Here's how the part is built. I have some questions about the finished solid (model axes, mm). Coordinates: 2 decimals unless noted, no trailing zeros. Write each loop counter-clockwise with the first axis right and the second up, starting at its lowest first coordinate (ties: lowest second). Pieces come first, ordered by that corner, then holes. Notation, with made-up numbers: (64.5, 74.5) -> (73.5, 74.5) arc R17 cw to (73.5, 78.5) -> close; hole circle Ø5 at (11.5, -13.75). An arc over 180 degrees is marked (long way). Use a Markdown table: item, result. Add a question column.
Autodesk Inventor part; units mm, degrees
ref_plane "YZ Plane" through (0, 0, 0) normal (1, 0, 0) x (0, 1, 0)
ref_plane "XZ Plane" through (0, 0, 0) normal (0, 1, 0) x (-1, 0, 0)
ref_plane "XY Plane" through (0, 0, 0) normal (0, 0, 1) x (1, 0, 0)
sketch "Sketch1" plane through (0, 0, 0) normal (0, 0, 1) x (1, 0, 0)
  line L0 (19.05, -25.4) -> (-19.05, -25.4)
  line L1 (-19.05, -25.4) -> (-19.05, 25.4)
  line L2 (-19.05, 25.4) -> (19.05, 25.4)
  line L3 (19.05, 25.4) -> (19.05, -25.4)
  line L4 (19.05, -25.4) -> (-19.05, 25.4) construction
  line L5 (-19.05, -25.4) -> (19.05, 25.4) construction
  point P0 (0, 0)
  dimension "d0" = 38.1
  dimension "d1" = 50.8
extrude "Extrusion1" add sketch "Sketch1" along normal blind 6.35
chamfer "Chamfer1" distance 12.7 angle 45 2 edges at (19.05, -25.4, 3.175) (-19.05, -25.4, 3.175)
sketch "Sketch2" plane through (0, 0, 6.35) normal (0, 0, 1) x (1, 0, 0)
  line L0 (-19.05, 25.4) -> (-19.05, -12.7) construction
  line L1 (19.05, -12.7) -> (19.05, 25.4) construction
  line L2 (-19.05, -12.7) -> (19.05, -12.7) construction
  line L3 (-6.35, -25.4) -> (6.35, -25.4) construction
  line L4 (0, -25.4) -> (0, 0) construction
  circle A0 centre (0, -12.7) radius 7.1
  circle A1 centre (0, -12.7) radius 17.5 construction
  circle A2 centre (-15.875, 0.635) radius 2.1
  circle A3 centre (-15.875, 13.335) radius 2
  circle A4 centre (15.875, 0.635) radius 2.1
  circle A5 centre (15.875, 13.335) radius 2
  dimension "d7" = 14.2
  dimension "d8" = 12.7
  dimension "d9" = 35
  dimension "d10" = 4.2
  dimension "d11" = 13.335
  dimension "d12" = 3.175
  dimension "d13" = 4
  dimension "d14" = 12.7
  dimension "d15" = 3.175
extrude "Extrusion2" cut sketch "Sketch2" against normal through all
properties part number "Lateral_Support_Connection2" material "Polystyrene"
Q1. Suppose I cut it at A-A, the plane x = 0. Write out the boundary of the cut face in (y, z), and give its area (3 significant figures).
Q2. Will these pins go through, and if not, where does the flat tip stop? pin 1 (2.5 mm diameter, centred on x = 15.875, y = 0.635, fed in from -Z); pin 2 (2 mm diameter, centred on x = -10.5, z = 1.5, fed in from -Y); pin 3 (3 mm diameter, centred on y = -19.5, z = 2.5, fed in from +X).
Q3. Thinking about a two-plate mould opening in Y: for faces 1 (the flat face through (0, -25.4, 3)), 2 (the cylindrical face through (14.3, 12.1, 3.2)), 3 (the flat face through (-19.05, 6, 3)), 4 (the cylindrical face through (-17.541, -0.643, 3.219)), which applies, released by +Y, released by -Y, zero draft, split by the parting line, or undercut?
Q4. Please list where these lines run through material, in increasing order: line 1 (X direction, y = 13, z = 5); line 2 (Y direction, x = 6, z = 5.75); line 3 (X direction, y = -10.5, z = 1.5).
Q5. Suppose I cut it at C-C, the plane x = -16.5. Write out the boundary of the cut face in (y, z), and give its area (3 significant figures).
Q6. Suppose I cut it at D-D, the plane z = 5.75. Write out the boundary of the cut face in (x, y) (3 decimals), and give its area (3 significant figures).
Q7. Suppose I cut it at B-B, the plane y = -14.5. Write out the boundary of the cut face in (x, z).
Answer key:
| question | item | result |
|---|---|---|
| 1 | outline | (-25.4, 0) -> (-19.8, 0) -> (-19.8, 6.35) -> (-25.4, 6.35) -> close; (-5.6, 0) -> (25.4, 0) -> (25.4, 6.35) -> (-5.6, 6.35) -> close |
| 1 | area | 232 mm^2 |
| 2 | pin 1 | passes through |
| 2 | pin 2 | stops at y = -22.25 |
| 2 | pin 3 | stops at x = 13.75 |
| 3 | face 1 | released by -Y |
| 3 | face 2 | undercut |
| 3 | face 3 | zero draft |
| 3 | face 4 | undercut |
| 4 | line 1 | x = -19.05 to -17.85, -13.9 to 13.9, 17.85 to 19.05 |
| 4 | line 2 | y = -25.4 to -16.5, -8.9 to 25.4 |
| 4 | line 3 | x = -19.05 to -6.75, 6.75 to 19.05 |
| 5 | outline | (-15.25, 0) -> (-1.37, 0) -> (-1.37, 6.35) -> (-15.25, 6.35) -> close; (2.64, 0) -> (11.44, 0) -> (11.44, 6.35) -> (2.64, 6.35) -> close; (15.23, 0) -> (25.4, 0) -> (25.4, 6.35) -> (15.23, 6.35) -> close |
| 5 | area | 209 mm^2 |
| 6 | outline | (-19.05, -12.7) -> (-6.35, -25.4) -> (6.35, -25.4) -> (19.05, -12.7) -> (19.05, 25.4) -> (-19.05, 25.4) -> close; hole circle Ø4.2 at (-15.875, 0.635); hole circle Ø4 at (-15.875, 13.335); hole circle Ø14.2 at (0, -12.7); hole circle Ø4.2 at (15.875, 0.635); hole circle Ø4 at (15.875, 13.335) |
| 6 | area | 1,560 mm^2 |
| 7 | outline | (-17.25, 0) -> (-6.87, 0) -> (-6.87, 6.35) -> (-17.25, 6.35) -> close; (6.87, 0) -> (17.25, 0) -> (17.25, 6.35) -> (6.87, 6.35) -> close |
